Design review of the part shown in the three views and the two pictorial views. Dimensions are in mm from the part's minimum x, y and z. Give positions to 0.01 mm unless a question says otherwise; leave off trailing zeros. Write each loop counter-clockwise with the first axis right and the second up, starting at its lowest first coordinate (ties: lowest second). Pieces come first, ordered by that corner, then holes. Notation, with made-up numbers: M 24.5,-24.75 L 67.5,-24.75 A28 ccw 67.5,1.25 Z; hole C 70.5,-35 d6. An arc over 180 degrees is marked long. Use one line per item in the form item = value. Start each with the question number.
Q1. For probe 1 along Y at (x, z) = (25, 3.35); probe 2 along Y at (x, z) = (7, 3.2); probe 3 along Y at (x, z) = (45, 3.7), list the stretches that pass through material, from the lowest coordinate up. Write a range as [from, to].
Q2. Consider section B-B on y = 46. Write out the cut boundary in (x, z).
Q3. Consider section C-C on z = 2.15. Write out the cut boundary in (x, y).
Q4. Consider section D-D on x = 34. Write out the cut boundary in (y, z).
Q5. Clearance check with a flat-ended pin moving along its axis: pin 1 Ø3 at (x, y) = (9.5, 43.5) entering from -Z. State where the tip first meets the part, or that it passes through.
Q6. Consider section A-A on x = 10. Write out the cut boundary in (y, z).
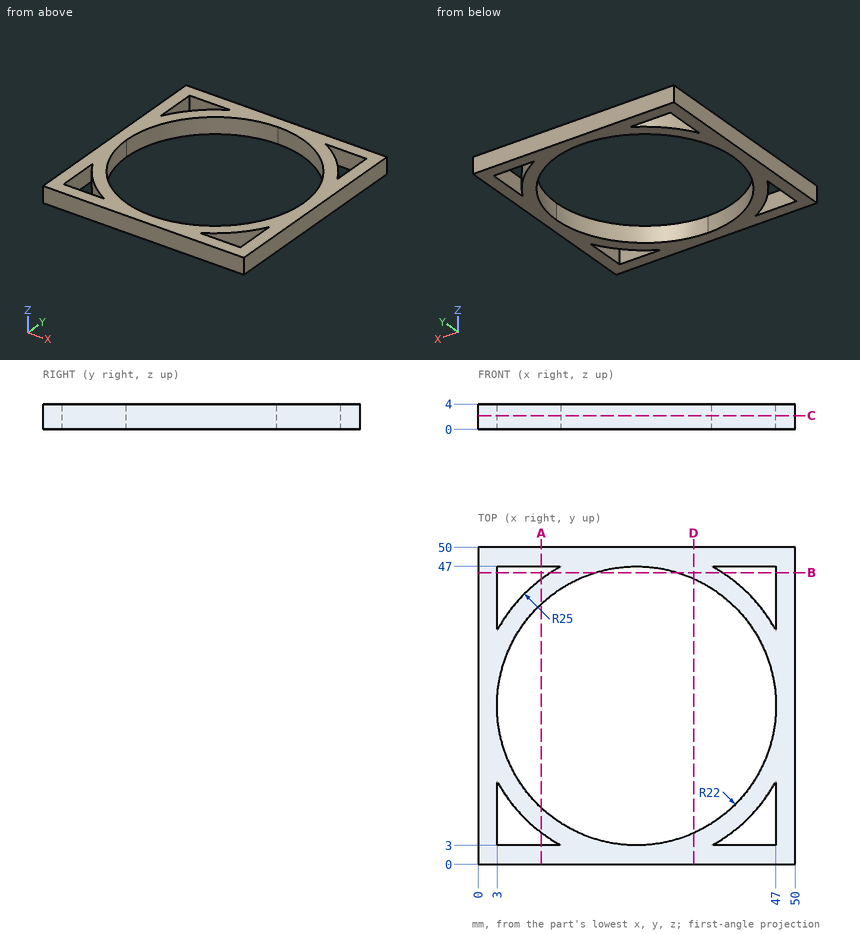
Working result:
q1.probe_1 = [0, 3], [47, 50]
q1.probe_2 = [0, 3], [7.65, 12.35], [37.65, 42.35], [47, 50]
q1.probe_3 = [0, 3], [10, 15.83], [34.17, 40], [47, 50]
q2.outline = M 0,0 L 3,0 L 3,4 L 0,4 Z; M 11.44,0 L 18.44,0 L 18.44,4 L 11.44,4 Z; M 31.56,0 L 38.56,0 L 38.56,4 L 31.56,4 Z; M 47,0 L 50,0 L 50,4 L 47,4 Z
q3.outline = M 0,0 L 50,0 L 50,50 L 0,50 Z; hole M 3,3 L 13.13,3 A25 cw 3,13.13 Z; hole C 25,25 d44; hole M 3,36.87 A25 cw 13.13,47 L 3,47 Z; hole M 36.87,3 L 47,3 L 47,13.13 A25 cw Z; hole M 36.87,47 A25 cw 47,36.87 L 47,47 Z
q4.outline = M 0,0 L 4.93,0 L 4.93,4 L 0,4 Z; M 45.07,0 L 50,0 L 50,4 L 45.07,4 Z
q5.pin_1 = 0
q6.outline = M 0,0 L 3,0 L 3,4 L 0,4 Z; M 5,0 L 8.91,0 L 8.91,4 L 5,4 Z; M 41.09,0 L 45,0 L 45,4 L 41.09,4 Z; M 47,0 L 50,0 L 50,4 L 47,4 Z
